Autodesk Inventor part; units mm, degrees
ref_plane "YZ Plane" through (0, 0, 0) normal (1, 0, 0) x (0, 1, 0)
ref_plane "XZ Plane" through (0, 0, 0) normal (0, 1, 0) x (-1, 0, 0)
ref_plane "XY Plane" through (0, 0, 0) normal (0, 0, 1) x (1, 0, 0)
sketch "Sketch1" plane through (0, 0, 0) normal (0, 1, 0) x (-1, 0, 0)
  line L0 (0, 0) -> (20, 0)
  line L1 (20, 0) -> (20, -20)
  line L2 (20, -20) -> (0, -20)
  line L3 (0, -20) -> (0, 0)
  circle A0 centre (14, -6.1) radius 2
  circle A1 centre (14, -13.9) radius 2
  dimension "d0" = 20
  dimension "d1" = 20
  dimension "d2" = 4
  dimension "d3" = 4
  dimension "d4" = 7.8
  dimension "d5" = 6.1
  dimension "d6" = 6
  dimension "d7" = 6
extrude "Extrusion1" add sketch "Sketch1" along normal blind 8
properties part number "motor spacer"
Geometry: final body of the model. Coordinates: model frame, mm. Give positions to 0.01 mm unless a question says otherwise; leave off trailing zeros. Order: outer loops, then holes, each group sorted by start corner. A loop starts at its lowest first (then second) coordinate and runs counter-clockwise, first axis right, second up. Notation, with made-up numbers: (69.25, 48) -> (84.25, 48) arc R13 ccw to (84.25, 70) -> close; hole circle Ø1 at (35, 73). An arc over 180 degrees is marked (long way). Write each question's results on one line, items separated by ' | '. Start each with the question number.
1) Section C-C (y = 5). Return loops of the section in (x, z).
2) Draft query along Z for faces 1 (the cylindrical face through (-12.4, 3.9, -4.9)), 2 (the flat face through (-10, 4, -20)), 3 (the flat face through (-20, 4, -10)). Return one class per face: pulls with the +Z half, pulls with the -Z half, needs draft (parallel to the pull), parting line crosses it, or undercut.
3) Section D-D (z = -13). Return loops of the section in (x, y).
4) Section A-A (x = -14). Return loops of the section in (y, z), then the cut area to 3 significant figures.
5) First-contact query: pin 1 (4.5 mm diameter, centred on x = -14, z = -13.9, fed in from -Y); pin 2 (2.5 mm diameter, centred on x = -14, z = -6.1, fed in from -Y). Flat tips, straight axial feed; report the tip coordinate or a pass-through.
6) Section B-B (z = -6.1). Return loops of the section in (x, y).
7) Line query: line 1 (Z direction, x = -14, y = 3.75); line 2 (X direction, y = 7, z = -14); line 3 (Z direction, x = -12.25, y = 7.25). Output: solid intervals per line, ascending. Write a range as from..to.
Calculated:
1) outline: (-20, -20) -> (0, -20) -> (0, 0) -> (-20, 0) -> close; hole circle Ø4 at (-14, -13.9); hole circle Ø4 at (-14, -6.1)
2) face 1: undercut | face 2: pulls with the -Z half | face 3: needs draft
3) outline: (-20, 0) -> (-15.79, 0) -> (-15.79, 8) -> (-20, 8) -> close; (-12.21, 0) -> (0, 0) -> (0, 8) -> (-12.21, 8) -> close
4) outline: (0, -20) -> (8, -20) -> (8, -15.9) -> (0, -15.9) -> close; (0, -11.9) -> (8, -11.9) -> (8, -8.1) -> (0, -8.1) -> close; (0, -4.1) -> (8, -4.1) -> (8, 0) -> (0, 0) -> close | area: 96.0 mm2
5) pin 1: y = 0 | pin 2: through
6) outline: (-20, 0) -> (-16, 0) -> (-16, 8) -> (-20, 8) -> close; (-12, 0) -> (0, 0) -> (0, 8) -> (-12, 8) -> close
7) line 1: -20..-15.9, -11.9..-8.1, -4.1..0 | line 2: -20..-16, -12..0 | line 3: -20..-14.87, -12.93..-7.07, -5.13..0
